from build123d import *

# Parameters (mm, degrees)
BOSS_EXTRUDE1_DEPTH  = 38.1
SKETCH5_W            = 76.2
SKETCH5_H            = 33.528
BOSS_EXTRUDE2_DEPTH  = 21.082
CUT_EXTRUDE2_DEPTH   = 88.66337421
SKETCH7_R            = 2.667
CUT_EXTRUDE3_DEPTH   = 69.500639142
SKETCH12_R           = 3.25
CUT_EXTRUDE7_DEPTH   = 2.54
SKETCH13_W           = 79.969594391
SKETCH13_H           = 52.20621733
CUT_EXTRUDE8_DEPTH   = 2.54
BOSS_EXTRUDE4_DEPTH  = 2.54
BOSS_EXTRUDE10_DEPTH = 2.54
FILLET8_R            = 1.27


with BuildPart() as part:
    # Sketch1 → Boss-Extrude1 (new, symmetric)
    with BuildSketch(Plane(origin=(0, 0, 0), x_dir=(0, 0, -1), z_dir=(1, 0, 0))):
        Polygon((0, 0), (33.528, 0), (14.297129242, 27.464529741), (0, 27.464529741), align=None)
    extrude(amount=BOSS_EXTRUDE1_DEPTH, both=True)

    # Sketch5 → Boss-Extrude2 (add)
    with BuildSketch(Plane.XZ):
        with Locations((0, -16.764)):
            Rectangle(SKETCH5_W, SKETCH5_H)
    extrude(amount=BOSS_EXTRUDE2_DEPTH)

    # Sketch6 → Cut-Extrude2 (cut, through all)
    with BuildSketch(Plane(origin=(38.1, 0, 0), x_dir=(0, 0, -1), z_dir=(1, 0, 0))):
        Polygon((2.54, 39.827095572), (2.54, -18.542), (30.427232545, -18.542), (30.427232545, 0), align=None)
    extrude(amount=-CUT_EXTRUDE2_DEPTH, mode=Mode.SUBTRACT)

    # Sketch7 → Cut-Extrude3 (cut, through all)
    with BuildSketch(Plane(origin=(0, -18.542, 0), x_dir=(1, 0, 0), z_dir=(0, 1, 0))):
        with Locations(Location((19.05, 15.24, 0), (0, 0, 270))):
            Circle(SKETCH7_R)
        with Locations(Location((-19.05, 15.24, 0), (0, 0, 270))):
            Circle(SKETCH7_R)
    extrude(amount=-CUT_EXTRUDE3_DEPTH, mode=Mode.SUBTRACT)

    # Sketch12 → Cut-Extrude7 (cut)
    with BuildSketch(Plane(origin=(0, 15.753007095, -22.497625683), x_dir=(-1, 0, 0), z_dir=(0, 0.5735764363510444, -0.8191520442889929))):
        with Locations(Location((0, -2.466870758, 0), (0, 0, 90))):
            Circle(SKETCH12_R)
    extrude(amount=-CUT_EXTRUDE7_DEPTH, mode=Mode.SUBTRACT)

    # Sketch13 → Cut-Extrude8 (cut)
    with BuildSketch(Plane.XY):
        with Locations((-0.230592833, 3.838694169)):
            Rectangle(SKETCH13_W, SKETCH13_H)
    extrude(amount=-CUT_EXTRUDE8_DEPTH, mode=Mode.SUBTRACT)

    # Sketch16 → Boss-Extrude4 (add)
    with BuildSketch(Plane(origin=(38.1, 0, 0), x_dir=(0, 0, -1), z_dir=(1, 0, 0))):
        Polygon((2.54, -18.542), (30.427232545, -18.542), (30.427232545, 0), (11.196361787, 27.464529741), align=None)
    extrude(amount=-BOSS_EXTRUDE4_DEPTH)

    # Sketch17 → Boss-Extrude10 (add)
    with BuildSketch(Plane.ZY.offset(38.1)):
        Polygon((-11.196361787, 27.464529741), (-30.427232545, 0), (-30.427232545, -18.542), (-2.54, -18.542), align=None)
    extrude(amount=-BOSS_EXTRUDE10_DEPTH)

    # Fillet8
    fillet8_edges = [part.edges().sort_by_distance(p)[0] for p in [
        (38.1, 13.73226487, -23.912564621),
        (38.1, 27.464529741, -12.746745514),
        (-38.1, -10.541, -33.528),
        (38.1, -10.541, -33.528),
        (0, -21.082, -33.528),
        (38.1, -21.082, -18.034),
        (-38.1, 27.464529741, -12.746745514),
        (-38.1, 13.73226487, -23.912564621),
        (0, 11.070020727, -25.776688039),
        (-38.1, -21.082, -18.034),
        (-38.1, -19.812, -2.54),
        (38.1, -19.812, -2.54),
        (0, 27.464529741, -14.297129242),
        (0, 0, -33.528),
        (35.56, -9.271, -30.427232545),
        (38.1, 4.46126487, -6.868180893),
        (0, -18.542, -30.427232545),
        (0, 0, -30.427232545),
        (-35.56, -9.271, -30.427232545),
        (-38.1, 4.46126487, -6.868180893),
    ]]
    fillet(fillet8_edges, radius=FILLET8_R)


solid = part.part
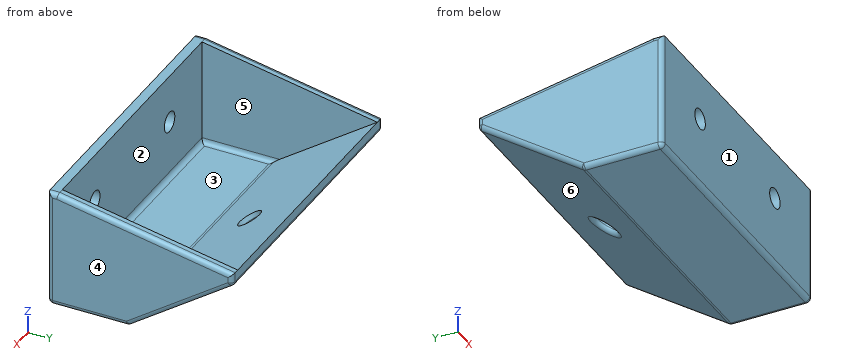
Verification items for the finished model (mm, model axes). Face numbers are marked on the shaded views. A direction names the side the tool comes from. Give positions to 0.01 mm unless a question says otherwise; leave off trailing zeros. Write each loop counter-clockwise with the first axis right and the second up, starting at its lowest first coordinate (ties: lowest second). Pieces come first, ordered by that corner, then holes.
(1) Material ranges on line 1 (X direction, y = -19.2, z = -15.24); line 2 (X direction, y = -16, z = -22); line 3 (Z direction, x = 19, y = -19), recorded low to high.
(2) Cross-section at B-B (x = 24). Enter the section's corners in (y, z), plus the area to 3 significant figures.
(3) Cross-section at A-A (x = -19.05). Enter the section's corners in (y, z), plus the area to 3 significant figures.
(4) Mould release check, pull along X, two halves, no side actions. Record for the marked faces 1, 2, 3 and 4: +X half, -X half, draft (parallel to the pull), parting line (faces both ways), or undercut.
(5) Gauge pin test, flat ends, axial feed: pin 1 (10 mm diameter, centred on x = -6.5, y = 4, fed in from +Z); pin 2 (2 mm diameter, centred on x = -10, y = 19, fed in from +Z); pin 3 (1.5 mm diameter, centred on x = -29.5, y = 6.5, fed in from -Z). Record the tip position at first contact, or that the pin passes through.
(6) Access from +Z, -Z, +X, -X, +Y, -Y to the whole of each face (thin tool, end or side, straight path). Record for the marked faces 5 and 6.
Worked out:
1. line 1: x = -38.1 to -21.72, -16.38 to 16.38, 21.72 to 38.1
1. line 2: x = -38.1 to -35.56, 35.56 to 38.1
1. line 3: z = -33.53 to -17.91, -12.57 to -2.54
2. outline: (-21.08, -32.26) arc R1.27 ccw to (-19.81, -33.53) - (-0.4, -33.53) arc R1.27 ccw to (0.33, -33.3) - (26.92, -14.68) arc R1.27 ccw to (27.46, -13.64) - (27.46, -11.2) - (0.33, -30.2) arc R1.27 cw to (-0.4, -30.43) - (-17.27, -30.43) arc R1.27 cw to (-18.54, -29.16) - (-18.54, -2.54) - (-21.08, -2.54) - close
2. area: 221 mm2
3. outline: (-21.08, -32.26) arc R1.27 ccw to (-19.81, -33.53) - (-0.4, -33.53) arc R1.27 ccw to (0.33, -33.3) - (26.92, -14.68) arc R1.27 ccw to (27.46, -13.64) - (27.46, -11.2) - (0.33, -30.2) arc R1.27 cw to (-0.4, -30.43) - (-17.27, -30.43) arc R1.27 cw to (-18.54, -29.16) - (-18.54, -17.91) - (-21.08, -17.91) - close; (-21.08, -12.57) - (-18.54, -12.57) - (-18.54, -2.54) - (-21.08, -2.54) - close
3. area: 208 mm2
4. face 1: draft
4. face 2: undercut
4. face 3: undercut
4. face 4: +X half
5. pin 1: stops at z = -24.13
5. pin 2: stops at z = -16.42
5. pin 3: stops at z = -29.5
6. face 5: +Z
6. face 6: -Z, +X, -X, +Y
